Source: CAD feature listing. Evaluate the final solid. Frame: model axes, mm. A direction names the side the tool comes from. Round coordinates to 2 decimals unless told otherwise and drop trailing zeros. Write each loop counter-clockwise with the first axis right and the second up, starting at its lowest first coordinate (ties: lowest second). Pieces come first, ordered by that corner, then holes. Notation, with made-up numbers: M 33,35.5 L 63,35.5 A13 cw 63,59.5 Z; hole C -14,66.25 d1. An arc over 180 degrees is marked long. Answer in a Markdown table with one row per item. Add a question column.
Item 1: Cut plane A-A on z = -13.5. Return loops of the section in (x, y), and give its area (3 significant figures).
Item 2: Contact query for flat-ended pins moving along their axis: pin 1 (2 mm diameter, centred on x = 7.5, z = 27.5, fed in from -Y); pin 2 (0.8 mm diameter, centred on y = 0.5, z = -30, fed in from +X); pin 3 (0.5 mm diameter, centred on x = 20.5, y = 0.5, fed in from -Z); pin 4 (14 mm diameter, centred on x = 4, z = 15.5, fed in from -Y). Output: stop coordinate, or through.
Item 3: Set-up query: faces 4 (the face through (42.43, 2.52, 42.4)), 5 (the face through (35, 3, -38)), 6 (the face through (0, 1, 13)). Return all of +Z, -Z, +X, -X, +Y, -Y with unobstructed straight access to the full face (end or side cutting, diameter ignored); none if empty.
Item 4: Mould query, pull axis Z, two halves, no side actions, for faces 1 (the face through (41.988, 0.382, 41.966)), 2 (the face through (-38, 3, -35)), 3 (the face through (-1, 0, -10)). Classes: released by +Z, released by -Z, zero draft, split by the parting line, or undercut.
Item 5: Cut plane C-C on z = -39. Return loops of the section in (x, y).
Item 6: Cut plane D-D on x = 2. Give the number of separate pieces and of enclosed holes in the cut face, and give its area (3 significant figures).
Item 7: Cut plane B-B on x = 21.5. Return loops of the section in (y, z), and give its area (3 significant figures).
Item 8: Material intervals for probe 1 along X at (y, z) = (2.5, -39); probe 2 along X at (y, z) = (1.5, 39); probe 3 along Z at (x, y) = (2, 2.15), sorted ascending.
from build123d import *

# Parameters (mm, degrees)
SKETCH_2_W           = 86
SKETCH_2_H           = 86
EXTRUDE_1_DEPTH      = 2
SKETCH_3_W           = 86
SKETCH_3_H           = 86
SKETCH_3_W_2         = 82
SKETCH_3_H_2         = 82
EXTRUDE_2_DEPTH      = 2
SKETCH_4_W           = 6
SKETCH_4_H           = 2
EXTRUDE_3_DEPTH      = 6
SKETCH_5_W           = 6
SKETCH_5_H           = 2
EXTRUDE_4_DEPTH      = 6
SKETCH_6_R           = 2.5
CUT_EXTRUDE_1_DEPTH  = 61.942595941
FILLET_1_R           = 2
CHAMFER_1_SIZE       = 1
SKETCH_7_W           = 28
SKETCH_7_H           = 28
CUT_EXTRUDE_2_DEPTH  = 1
SKETCH_8_R           = 1.25
SKETCH_8_W           = 19
SKETCH_8_H           = 3
CUT_EXTRUDE_10_DEPTH = 61.88513776
SKETCH_9_W           = 6
SKETCH_9_H           = 6
CUT_EXTRUDE_11_DEPTH = 61.942595941
CHAMFER_2_SIZE       = 1
CHAMFER_3_SIZE       = 1


with BuildPart() as part:
    # 草图2 → 凸台-拉伸1 (new body)
    with BuildSketch(Plane(origin=(0, 0, 0), x_dir=(1, 0, 0), z_dir=(0, 1, 0))):
        Rectangle(SKETCH_2_W, SKETCH_2_H)
    extrude(amount=EXTRUDE_1_DEPTH)

    # 草图3 → 凸台-拉伸2 (add)
    with BuildSketch(Plane(origin=(0, 2, 0), x_dir=(1, 0, 0), z_dir=(0, 1, 0))):
        Rectangle(SKETCH_3_W, SKETCH_3_H)
        Rectangle(SKETCH_3_W_2, SKETCH_3_H_2, mode=Mode.SUBTRACT)
    extrude(amount=EXTRUDE_2_DEPTH)

    # 草图4 → 凸台-拉伸3 (add)
    with BuildSketch(Plane(origin=(0, 0, 41), x_dir=(-1, 0, 0), z_dir=(0, 0, -1))):
        with Locations((-38, 3)):
            Rectangle(SKETCH_4_W, SKETCH_4_H)
        with Locations((38, 3)):
            Rectangle(SKETCH_4_W, SKETCH_4_H)
    extrude(amount=EXTRUDE_3_DEPTH)

    # 草图5 → 凸台-拉伸4 (add)
    with BuildSketch(Plane.XY.offset(-41)):
        with Locations((-38, 3)):
            Rectangle(SKETCH_5_W, SKETCH_5_H)
        with Locations((38, 3)):
            Rectangle(SKETCH_5_W, SKETCH_5_H)
    extrude(amount=EXTRUDE_4_DEPTH)

    # 草图6 → 切除-拉伸1 (cut, through all)
    with BuildSketch(Plane(origin=(0, 4, 0), x_dir=(1, 0, 0), z_dir=(0, 1, 0))):
        with Locations(Location((-39, 39, 0), (0, 0, 270))):
            Circle(SKETCH_6_R)
        with Locations(Location((39, 39, 0), (0, 0, 90))):
            Circle(SKETCH_6_R)
        with Locations(Location((39, -39, 0), (0, 0, 270))):
            Circle(SKETCH_6_R)
        with Locations(Location((-39, -39, 0), (0, 0, 90))):
            Circle(SKETCH_6_R)
    extrude(amount=-CUT_EXTRUDE_1_DEPTH, mode=Mode.SUBTRACT)

    # 圆角1
    fillet_1_edges = [part.edges().sort_by_distance(p)[0] for p in [
        (43, 2, 43),
        (-43, 2, 43),
        (-43, 2, -43),
        (43, 2, -43),
    ]]
    fillet(fillet_1_edges, radius=FILLET_1_R)

    # 倒角1
    chamfer_1_edges = [part.edges().sort_by_distance(p)[0] for p in [
        (-43, 0, 0),
        (43, 0, 0),
        (0, 0, 43),
        (0, 0, -43),
        (42.414213562, 0, -42.414213562),
        (42.414213562, 0, 42.414213562),
        (-42.414213562, 0, 42.414213562),
        (-42.414213562, 0, -42.414213562),
    ]]
    chamfer(chamfer_1_edges, length=CHAMFER_1_SIZE)

    # 草图7 → 切除-拉伸2 (cut)
    with BuildSketch(Plane.XZ):
        with Locations((0, 13)):
            Rectangle(SKETCH_7_W, SKETCH_7_H)
    extrude(amount=-CUT_EXTRUDE_2_DEPTH, mode=Mode.SUBTRACT)

    # 草图8 → 切除-拉伸10 (cut, through all)
    with BuildSketch(Plane.XZ.offset(-1)):
        with Locations(Location((-11.7, 24.382645166, 0), (0, 0, 270))):
            Circle(SKETCH_8_R)
        with Locations(Location((11.7, 24.382645166, 0), (0, 0, 270))):
            Circle(SKETCH_8_R)
        with Locations(Location((-11.7, 1, 0), (0, 0, 270))):
            Circle(SKETCH_8_R)
        with Locations(Location((11.7, 1, 0), (0, 0, 270))):
            Circle(SKETCH_8_R)
        with Locations((0, 24.382645166)):
            Rectangle(SKETCH_8_W, SKETCH_8_H)
    extrude(amount=-CUT_EXTRUDE_10_DEPTH, mode=Mode.SUBTRACT)

    # 草图9 → 切除-拉伸11 (cut, through all)
    with BuildSketch(Plane.XZ):
        with Locations((0, -14)):
            Rectangle(SKETCH_9_W, SKETCH_9_H)
        with Locations((-20, -14)):
            Rectangle(SKETCH_9_W, SKETCH_9_H)
        with Locations((20, -14)):
            Rectangle(SKETCH_9_W, SKETCH_9_H)
        with Locations((-20, -29)):
            Rectangle(SKETCH_9_W, SKETCH_9_H)
        with Locations((0, -29)):
            Rectangle(SKETCH_9_W, SKETCH_9_H)
        with Locations((20, -29)):
            Rectangle(SKETCH_9_W, SKETCH_9_H)
    extrude(amount=-CUT_EXTRUDE_11_DEPTH, mode=Mode.SUBTRACT)

    # 倒角2
    chamfer_2_edges = [part.edges().sort_by_distance(p)[0] for p in [
        (-3, 2, -29),
        (0, 2, -26),
        (3, 2, -29),
        (0, 2, -32),
        (20, 2, -26),
        (23, 2, -29),
        (20, 2, -32),
        (17, 2, -29),
        (-20, 2, -26),
        (-17, 2, -29),
        (-20, 2, -32),
        (-23, 2, -29),
    ]]
    chamfer(chamfer_2_edges, length=CHAMFER_2_SIZE)

    # 倒角3
    chamfer_3_edges = [part.edges().sort_by_distance(p)[0] for p in [
        (17, 2, -14),
        (20, 2, -11),
        (23, 2, -14),
        (20, 2, -17),
        (-23, 2, -14),
        (-20, 2, -11),
        (-17, 2, -14),
        (-20, 2, -17),
        (-3, 2, -14),
        (0, 2, -11),
        (3, 2, -14),
        (0, 2, -17),
    ]]
    chamfer(chamfer_3_edges, length=CHAMFER_3_SIZE)


solid = part.part
Results below:
| question | item | result |
|---|---|---|
| 1 | outline | M -43,1 L -42,0 L -23,0 L -23,1 L -24,2 L -41,2 L -41,4 L -43,4 Z; M -17,0 L -3,0 L -3,1 L -4,2 L -16,2 L -17,1 Z; M 3,0 L 17,0 L 17,1 L 16,2 L 4,2 L 3,1 Z; M 23,0 L 42,0 L 43,1 L 43,4 L 41,4 L 41,2 L 24,2 L 23,1 Z |
| 1 | area | 140 mm2 |
| 2 | pin 1 | y = 0 |
| 2 | pin 2 | x = 42.9 |
| 2 | pin 3 | z = -42.75 |
| 2 | pin 4 | y = 1 |
| 3 | face 4 | +Z, +X, +Y, -Y |
| 3 | face 5 | +Y |
| 3 | face 6 | -Y |
| 4 | face 1 | released by +Z |
| 4 | face 2 | undercut |
| 4 | face 3 | zero draft |
| 5 | outline | M -43,1 L -42,0 L -41.5,0 L -41.5,4 L -43,4 Z; M -36.5,0 L 36.5,0 L 36.5,4 L 35,4 L 35,2 L -35,2 L -35,4 L -36.5,4 Z; M 41.5,0 L 42,0 L 43,1 L 43,4 L 41.5,4 Z |
| 6 | separate pieces | 4 |
| 6 | enclosed holes | 0 |
| 6 | area | 122 mm2 |
| 7 | outline | M 0,-42 L 1,-43 L 4,-43 L 4,-41 L 2,-41 L 2,-33 L 1,-32 L 0,-32 Z; M 0,-26 L 1,-26 L 2,-25 L 2,-18 L 1,-17 L 0,-17 Z; M 0,-11 L 1,-11 L 2,-10 L 2,41 L 4,41 L 4,43 L 1,43 L 0,42 Z |
| 7 | area | 153 mm2 |
| 8 | probe 1 | -43 to -41.5, -36.5 to -35, 35 to 36.5, 41.5 to 43 |
| 8 | probe 2 | -43 to -41.5, -36.5 to 36.5, 41.5 to 43 |
| 8 | probe 3 | -43 to -41, 41 to 43 |
